The model under review builds one solid part; all positions refer to its coordinate system, in mm. Face numbers are marked on the shaded views. A direction names the side the tool comes from. Give positions to 0.01 mm unless a question says otherwise; leave off trailing zeros. Write each loop counter-clockwise with the first axis right and the second up, starting at its lowest first coordinate (ties: lowest second). Pieces come first, ordered by that corner, then holes.
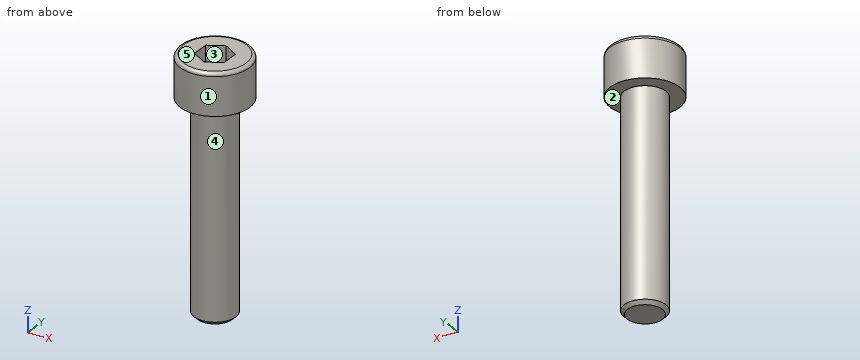
from build123d import *

# Parameters (mm, degrees)
ESQUISSE1_R             = 3
BASE_EXTRUSION_DEPTH    = 36
CHANFREIN1_SIZE         = 0.5
ESQUISSE2_R             = 5
BOSS_EXTRU_1_DEPTH      = 6
ENL_V_MAT_EXTRU_1_DEPTH = 3.5
CONG_2_R                = 0.5


with BuildPart() as part:
    # Esquisse1 → Base-Extrusion (new body)
    with BuildSketch(Plane.XY):
        Circle(ESQUISSE1_R)
    extrude(amount=BASE_EXTRUSION_DEPTH)

    # Chanfrein1
    chanfrein1_edges = [part.edges().sort_by_distance(p)[0] for p in [
        (-3, 0, 0),
    ]]
    chamfer(chanfrein1_edges, length=CHANFREIN1_SIZE)

    # Esquisse2 → Boss.-Extru.1 (add)
    with BuildSketch(Plane.XY.offset(30)):
        Circle(ESQUISSE2_R)
    extrude(amount=BOSS_EXTRU_1_DEPTH)

    # Esquisse3 → Enlèv. mat.-Extru.1 (cut)
    with BuildSketch(Plane.XY.offset(36)):
        Polygon((0, 2.5), (-2.165063509, 1.25), (-2.165063509, -1.25), (0, -2.5), (2.165063509, -1.25), (2.165063509, 1.25), align=None)
    extrude(amount=-ENL_V_MAT_EXTRU_1_DEPTH, mode=Mode.SUBTRACT)

    # Congé2
    cong_2_edges = [part.edges().sort_by_distance(p)[0] for p in [
        (-5, 0, 36),
    ]]
    fillet(cong_2_edges, radius=CONG_2_R)


solid = part.part
1) Consider section C-C, the plane z = 26.5. Give the boundary of the cut face in (x, y), then the cut area to 3 significant figures.
2) Consider section A-A, the plane z = 33. Give the boundary of the cut face in (x, y).
3) Tool access review of the marked faces 4 and 5: name each direction out of +Z, -Z, +X, -X, +Y, -Y from which nothing blocks a thin tool from reaching the whole face with its end or side.
4) Insertion check: pin 1 (6 mm diameter, centred on x = 1.5, z = 25.5, fed in from +Y); pin 2 (5 mm diameter, centred on y = 0.5, z = 11, fed in from +X); pin 3 (1.5 mm diameter, centred on x = -1.5, z = 12.5, fed in from +Y). Each pin has a flat end and moves straight along its axis. Give the tip position at first contact, or say it passes through.
5) The part is to be moulded in two halves that separate along Y. For the marked faces 1, 2 and 3, say which applies: +Y half, -Y half, draft (parallel to the pull), parting line (faces both ways), or undercut.
6) To check wall thickness, follow probe 1 along Z at (x, y) = (2.5, -3.5); probe 2 along Z at (x, y) = (-0.25, 0.25); probe 3 along Y at (x, z) = (0.25, 5). State the ranges of each line that lie inside material, in increasing order.
7) Consider section B-B, the plane y = 0. Give the boundary of the cut face in (x, z), then the cut area to 3 significant figures.
Answer block:
1. outline: circle Ø6 at (0, 0)
1. area: 28.3 mm2
2. outline: circle Ø10 at (0, 0); hole (-2.17, -1.25) - (0, -2.5) - (2.17, -1.25) - (2.17, 1.25) - (0, 2.5) - (-2.17, 1.25) - close
3. face 4: -Z
3. face 5: +Z, +X, -X, +Y, -Y
4. pin 1: stops at y = 3
4. pin 2: stops at x = 3
4. pin 3: stops at y = 2.9
5. face 1: parting line
5. face 2: draft
5. face 3: undercut
6. probe 1: z = 30 to 36
6. probe 2: z = 0 to 32.5
6. probe 3: y = -2.99 to 2.99
7. outline: (-5, 30) - (-3, 30) - (-3, 0.5) - (-2.5, 0) - (2.5, 0) - (3, 0.5) - (3, 30) - (5, 30) - (5, 35.5) arc R0.5 ccw to (4.5, 36) - (2.17, 36) - (2.17, 32.5) - (-2.17, 32.5) - (-2.17, 36) - (-4.5, 36) arc R0.5 ccw to (-5, 35.5) - close
7. area: 224 mm2
